Geometry: see drawing. Coordinates: mm, zero at the bounding-box minimum. Coordinates: 2 decimals unless noted, no trailing zeros. Write each loop counter-clockwise with the first axis right and the second up, starting at its lowest first coordinate (ties: lowest second). Pieces come first, ordered by that corner, then holes. Notation, with made-up numbers: (17.25, -25) - (42.25, -25) arc R22 ccw to (42.25, 6) - close; hole circle Ø10 at (2.25, -2). An arc over 180 degrees is marked (long way). Use a Markdown table: item, result. Add a question column.
Q1. Section query B-B (z = 500). Return the cut outline in (x, y).
Q2. Mould query, pull axis X, two halves, no side actions, for the marked faces 1 and 2. Classes: released by +X, released by -X, zero draft, split by the parting line, or undercut.
Q3. Section query A-A (x = 93.5). Return the cut outline in (y, z).
Q4. Material intervals for probe 1 along X at (y, z) = (6, 575); probe 2 along Y at (x, z) = (190, 493); probe 3 along Y at (x, z) = (20.5, 422.5), sorted ascending. Write a range as from..to.
Q5. Pin query (flat end, axial travel): P1, Ø3, axis at x = 150, z = 166.5, coming from the -Y side; P2, Ø1.5, axis at x = 161.5, z = 301.5, coming from the +Y side; P3, Ø3, axis at y = 36.5, z = 222, coming from the +X side. Return the tip coordinate at first contact, or that it passes through.
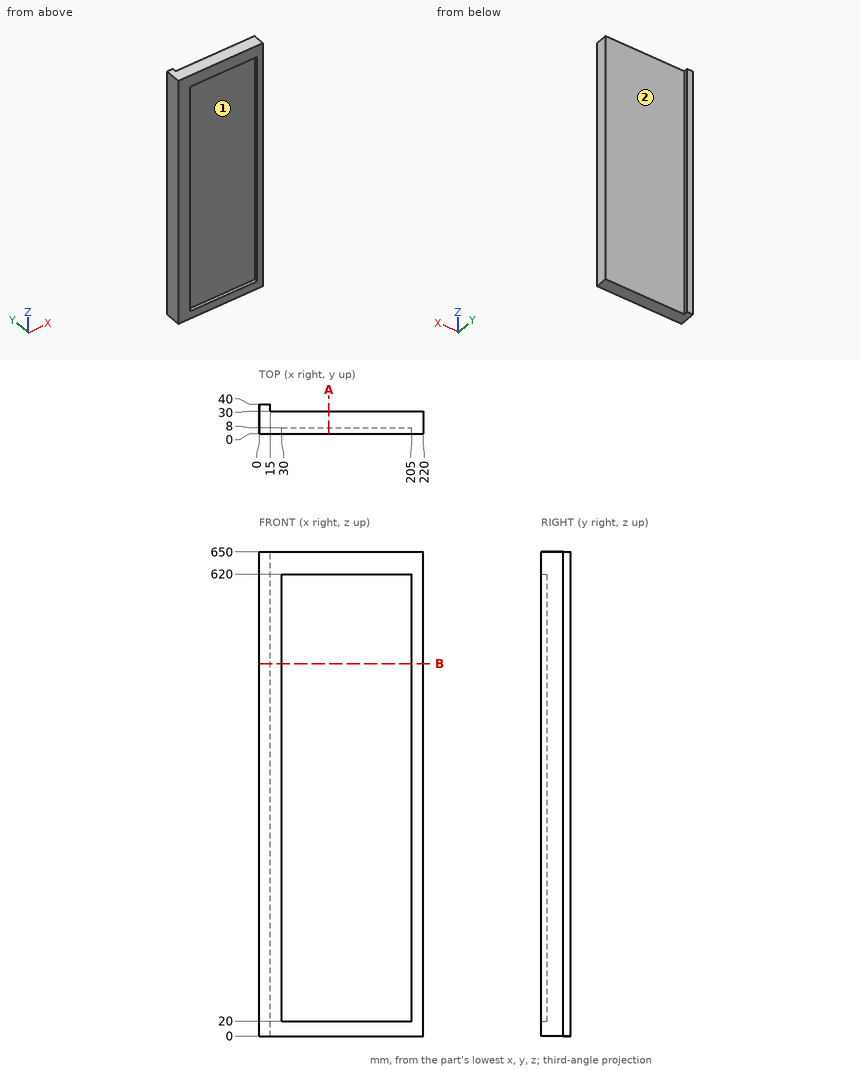
Values follow:
| question | item | result |
|---|---|---|
| 1 | outline | (0, 0) - (30, 0) - (30, 8) - (205, 8) - (205, 0) - (220, 0) - (220, 30) - (15, 30) - (15, 40) - (0, 40) - close |
| 2 | face 1 | undercut |
| 2 | face 2 | zero draft |
| 3 | outline | (0, 0) - (30, 0) - (30, 650) - (0, 650) - (0, 620) - (8, 620) - (8, 20) - (0, 20) - close |
| 4 | probe 1 | 0..30, 205..220 |
| 4 | probe 2 | 8..30 |
| 4 | probe 3 | 0..30 |
| 5 | P1 | y = 8 |
| 5 | P2 | y = 30 |
| 5 | P3 | x = 15 |
